Autodesk Inventor part; units mm, degrees
ref_plane "YZ Plane" through (0, 0, 0) normal (1, 0, 0) x (0, 1, 0)
ref_plane "XZ Plane" through (0, 0, 0) normal (0, 1, 0) x (-1, 0, 0)
ref_plane "XY Plane" through (0, 0, 0) normal (0, 0, 1) x (1, 0, 0)
sketch "Sketch1" plane through (0, 0, 0) normal (0, 1, 0) x (-1, 0, 0)
  line L0 (0, 0) -> (-3.16, 0)
  line L1 (-3.16, 0) -> (-2.16, -1)
  line L2 (-2.16, -1) -> (-2.16, -2.701)
  arc A0 (-2.16, -2.701) -> (-0.6835, -4.75) centre (0, -2.701) ccw
  line L3 (0, -5.6986) -> (0, -8.55)
  line L4 (-1, -9.55) -> (-3.65, -9.55)
  line L5 (-4.65, -8.55) -> (-4.65, -5.75)
  line L6 (-5.65, -4.75) -> (-5.85, -4.75)
  line L7 (-5.85, -4.75) -> (-6.85, -3.75)
  line L8 (-6.85, -3.75) -> (-6.85, -1)
  line L9 (-6.85, -1) -> (-5.85, 0)
  line L10 (-5.85, 0) -> (-3.16, 0)
  circle A1 centre (-4.505, -2.1243) radius 1.45
  circle A2 centre (-2.305, -7.1243) radius 1.45
  arc A3 (0, -5.6986) -> (-0.6835, -4.75) centre (-1, -5.6986) ccw
  arc A4 (-4.65, -5.75) -> (-5.65, -4.75) centre (-5.65, -5.75) ccw
  arc A5 (-1, -9.55) -> (0, -8.55) centre (-1, -8.55) ccw
  arc A6 (-4.65, -8.55) -> (-3.65, -9.55) centre (-3.65, -8.55) ccw
  point P0 (0, -4.861)
  point P1 (-4.65, -7.15)
  point P2 (-4.505, 0)
  point P3 (-5.75, -4.75)
  point P4 (0, -7.1243)
  dimension "d0" = 5
  dimension "d1" = 2.2
  dimension "d2" = 2.9
  dimension "d3" = 4.75
  dimension "d4" = 4.65
  dimension "d6" = 4.69
  dimension "d8" = 6.85
  dimension "d9" = 9.55
  dimension "d10" = 135
  dimension "d11" = 135
  dimension "d12" = 135
  dimension "d13" = 1
  dimension "d14" = 1
  dimension "d70" = 2.75
extrude "Extrusion1" add sketch "Sketch1" along normal blind 1.8 contours L1 L2 A0 A3 L3 A5 L4 A6 L5 A4 L6 L7 L8 L9 L10 | A1 | A2
extrude "Extrusion2" add sketch "Sketch1" against normal blind 1.25 contours A1 | A2
chamfer "Chamfer1" distance 0.1 angle 45 2 edges at (5.955, -1.25, -2.1243) (3.755, -1.25, -7.1243)
sketch "Sketch2" plane through (3.16, 0, 0) normal (0, 0, 1) x (1, 0, 0)
  line L0 (1.49, 1.8) -> (2.49, 1.8)
  line L1 (2.185, -0.05) -> (0.505, -0.05)
  line L2 (0.49, 0) -> (0.49, 1.8)
  line L3 (2.69, 0) -> (2.69, 1.8)
  line L4 (0, 0) -> (0, 1.8)
  line L5 (0, 1.8) -> (2.69, 1.8)
  line L6 (2.185, -0.05) -> (2.185, 1.7)
  line L7 (0.505, -0.05) -> (0.505, 1.7)
  line L8 (0.605, 1.7) -> (0.605, 0.05)
  line L9 (0.605, 0.05) -> (2.085, 0.05)
  line L10 (2.085, 0.05) -> (2.085, 1.7)
  line L11 (2.185, 1.7) -> (2.085, 1.7)
  line L12 (0.605, 1.7) -> (0.505, 1.7)
  point P0 (-3.16, 0)
  dimension "d24" = 1.68
  dimension "d26" = 1.85
  dimension "d27" = 0.1
  dimension "d28" = 0.505
  dimension "d29" = 0.505
  dimension "d30" = 0.1
  dimension "d31" = 0.1
extrude "Extrusion3" add sketch "Sketch2" along normal blind 1.8
sketch "Sketch3" plane through (3.665, 0, 0) normal (-1, 0, 0) x (0, 0, 1)
  line L0 (0, -0.05) -> (1.8, -0.05)
  line L1 (0.16, -0.05) -> (0.16, 0.54)
  line L2 (0, 0) -> (0, 1.7)
  arc A0 (0.16, 0.54) -> (0, 0.7) centre (0, 0.54) ccw
  line L3 (0, 0) -> (0, 1.8)
  line L4 (0, 0) -> (0, 1.7)
  line L5 (0, 0) -> (0, -0.05)
  line L6 (0, -0.05) -> (1.8, -0.05)
  line L7 (1.8, 1.7) -> (1.8, -0.05)
  line L8 (0, 1.7) -> (1.8, 1.7)
  point P0 (0, 0)
  point P1 (0, -0.05)
  dimension "d34" = 0.16
  dimension "d54" = 0.75
extrude "Extrusion4" cut sketch "Sketch3" against normal through all contours L5 L2 A0 L1 L0
sketch "Sketch4" plane through (3.65, 0, -9.55) normal (0, 0, -1) x (-1, 0, 0)
  line L0 (2.165, -0.05) -> (0.485, -0.05)
  line L1 (2.165, -0.05) -> (2.165, 1.7)
  line L2 (0.485, -0.05) -> (0.485, 1.7)
  line L3 (0.585, 1.7) -> (0.585, 0.05)
  line L4 (0.585, 0.05) -> (2.065, 0.05)
  line L5 (2.065, 0.05) -> (2.065, 1.7)
  line L6 (2.165, 1.7) -> (2.065, 1.7)
  line L7 (0.585, 1.7) -> (0.485, 1.7)
  line L8 (2.65, 0) -> (2.65, 1.8)
  line L9 (0, 1.8) -> (2.65, 1.8)
  line L10 (0, 0) -> (0, 1.8)
  point P0 (3.65, 0)
  dimension "d37" = 1.68
  dimension "d42" = 0.1
  dimension "d43" = 0.1
  dimension "d44" = 0.485
  dimension "d45" = 0.485
  dimension "d46" = 1.85
  dimension "d47" = 0.1
extrude "Extrusion5" add sketch "Sketch4" along normal blind 1.8
sketch "Sketch5" plane through (1.485, 0, -9.55) normal (-1, 0, 0) x (0, 0, 1)
  line L0 (0, -0.05) -> (0, 0)
  line L1 (0, 1.7) -> (0, 0)
  line L2 (0, 1.7) -> (-1.8, 1.7)
  line L3 (-1.8, -0.05) -> (-1.8, 1.7)
  line L4 (0, -0.05) -> (-1.8, -0.05)
  line L5 (-0.16, -0.05) -> (-0.16, 0.54)
  arc A0 (0, 0.7) -> (-0.16, 0.54) centre (0, 0.54) ccw
  point P0 (9.55, 0)
  point P1 (-1.867, -0.613)
  point P2 (-1.867, -0.6608)
  point P3 (0, -0.025)
  dimension "d51" = 0.16
  dimension "d55" = 0.75
extrude "Extrusion6" cut sketch "Sketch5" against normal through all contours L4 L5 A0 L1 L0
sketch "Sketch6" plane through (4.505, -1.25, -2.1243) normal (0, -1, 0) x (1, 0, 0)
  line L0 (0.1, 0.6) -> (-0.1, 0.6)
  line L1 (-0.1, 0.6) -> (-0.1, -0.6)
  line L2 (-0.1, -0.6) -> (0.1, -0.6)
  line L3 (0.1, -0.6) -> (0.1, 0.6)
  line L4 (-2.1, -4.4) -> (-2.3, -4.4)
  line L5 (-2.3, -4.4) -> (-2.3, -5.6)
  line L6 (-2.3, -5.6) -> (-2.1, -5.6)
  line L7 (-2.1, -5.6) -> (-2.1, -4.4)
  circle A0 centre (0, 0) radius 1.35
  circle A1 centre (-2.2, -5) radius 1.35
  point P0 (-4.505, 2.1243)
  point P1 (0.1, 0)
  point P2 (0, 0.6)
  point P3 (-2.1, -5)
  point P4 (-2.2, -4.4)
  dimension "d56" = 1.2
  dimension "d57" = 0.2
  dimension "d58" = 1.2
  dimension "d59" = 0.2
extrude "Extrusion7" cut sketch "Sketch6" against normal through all contours L3 L2 L1 L0 | L7 L6 L5 L4
chamfer "Chamfer2" distance 0.2 angle 45 8 edges at (4.605, -1.25, -2.1243) (4.505, -1.25, -1.5243) (4.405, -1.25, -2.1243) (4.505, -1.25, -2.7243) (2.405, -1.25, -7.1243) (2.305, -1.25, -6.5243) (2.205, -1.25, -7.1243) (2.305, -1.25, -7.7243)
fillet "Fillet1" radius 0.4 8 edges at (3.665, -0.05, 0.98) (5.345, -0.05, 0.98) (5.245, 0.05, 0.98) (3.765, 0.05, 0.98) (1.485, -0.05, -10.53) (3.165, -0.05, -10.53) (3.065, 0.05, -10.53) (1.585, 0.05, -10.53)
sketch "Sketch7" plane through (4.065, -0.05, 1.8) normal (0, -1, 0) x (1, 0, 0)
  line L0 (0.24, 0) -> (0.64, 0)
  line L1 (0.64, 0) -> (0.64, -1.64)
  line L2 (0.64, -1.64) -> (0.24, -1.64)
  line L3 (0.24, -1.64) -> (0.24, 0)
  line L4 (0, 0) -> (0.88, 0)
  line L5 (-1.94, -11.51) -> (-1.54, -11.51)
  line L6 (-1.54, -11.51) -> (-1.54, -13.15)
  line L7 (-1.54, -13.15) -> (-1.94, -13.15)
  line L8 (-1.94, -13.15) -> (-1.94, -11.51)
  line L9 (-1.3, -11.51) -> (-2.18, -11.51)
  line L10 (-1.3, -13.15) -> (-2.18, -13.15)
  line L11 (0, -1.64) -> (0.88, -1.64)
  point P0 (-4.065, -1.8)
  point P1 (0.44, 0)
  point P2 (0.44, 0)
  point P3 (-1.74, -11.51)
  point P4 (-1.74, -11.51)
  dimension "d66" = 0.4
  dimension "d67" = 0.4
extrude "Extrusion8" cut sketch "Sketch7" against normal through all
equation "\"d11\" = d10"
equation "\"d29\" = d28"
properties part number "Kailh Choc Hotswap Socket"
Design review of the part built by this model. Coordinates are the model's own, in mm. A direction names the side the tool comes from. Give positions to 0.01 mm unless a question says otherwise; leave off trailing zeros. Write each loop counter-clockwise with the first axis right and the second up, starting at its lowest first coordinate (ties: lowest second). Pieces come first, ordered by that corner, then holes.
(1) Clearance check with flat-ended pins moving along their axes: pin 1 Ø0.9 at (y, z) = (1, -1.5) entering from -X; pin 2 Ø1.4 at (y, z) = (1, 1) entering from -X (3 decimals); pin 3 Ø0.6 at (x, y) = (2, 0) entering from +Z. State where each tip first meets the part, or that it passes through.
Checked values:
pin 1: stops at x = 2.16
pin 2: stops at x = 3.665
pin 3: stops at z = -0.86
(2) Wall thickness on line 1 along X through (y, z) = (0.8, -7.25) (3 decimals); line 2 along Y through (x, z) = (6, -3.25); line 3 along Z through (x, y) = (5.75, 0.75): over which ranges is each line inside the solid? List them lowest first.
Checked values:
line 1: x = 0 to 2.205, 2.405 to 4.65
line 2: y = 0 to 1.8
line 3: z = -4.75 to 0
(3) Add section B-B (y = -0.2). Give the boundary of the cut face in (x, z) (3 decimals).
Checked values:
outline: circle Ø2.9 at (2.305, -7.124); circle Ø2.9 at (4.505, -2.124); hole (2.205, -7.724) - (2.405, -7.724) - (2.405, -6.524) - (2.205, -6.524) - close; hole (4.405, -2.724) - (4.605, -2.724) - (4.605, -1.524) - (4.405, -1.524) - close
(4) Add section A-A (z = -10.25). Give the boundary of the cut face in (x, y) (3 decimals), and give its area (3 significant figures).
Checked values:
outline: (1.485, 0.35) arc R0.4 ccw to (1.885, -0.05) - (2.125, -0.05) - (2.125, 0.05) - (1.985, 0.05) arc R0.4 cw to (1.585, 0.45) - (1.585, 1.7) - (1.485, 1.7) - close; (2.525, -0.05) - (2.765, -0.05) arc R0.4 ccw to (3.165, 0.35) - (3.165, 1.7) - (3.065, 1.7) - (3.065, 0.45) arc R0.4 cw to (2.665, 0.05) - (2.525, 0.05) - close
area: 0.458 mm2
(5) Add section D-D (z = -5.5). Give the boundary of the cut face in (x, y).
Checked values:
outline: (0.02, 0) - (4.68, 0) - (4.68, 1.8) - (0.02, 1.8) - close
(6) Tool access review of faces 1 (the face through (2.16, 1, -2)), 2 (the face through (0.285, 0.887, -9.249)), 3 (the face through (2.405, 0, -7)), 4 (the face through (3, 0, -5)), 5 (the face through (6.36, 0.89, -0.51)): name each direction out of +Z, -Z, +X, -X, +Y, -Y from which nothing blocks a thin tool from reaching the whole face with its end or side.
Checked values:
face 1: +Z, -X, +Y, -Y
face 2: -Z, -X, +Y, -Y
face 3: +Y, -Y
face 4: -Y
face 5: +Z, +X, +Y, -Y
(7) Mouldability with a two-part tool opening along X and no side actions: class faces 6 (the face through (5, 1, 0)), 7 (the face through (6.3, 0.9, -4.3)), 8 (the face through (1.74, 0.89, -3.98)) as +X half, -X half, draft (parallel to the pull), parting line (faces both ways), or undercut.
Checked values:
face 6: undercut
face 7: +X half
face 8: -X half
(8) Add section C-C (y = 1.4). Give the number of separate pieces and of enclosed holes in the cut face, and give its area (3 significant figures).
Checked values:
separate pieces: 1
enclosed holes: 2
area: 43.8 mm2
